Autodesk Inventor part; units mm, degrees
ref_plane "YZ Plane" through (0, 0, 0) normal (1, 0, 0) x (0, 1, 0)
ref_plane "XZ Plane" through (0, 0, 0) normal (0, 1, 0) x (-1, 0, 0)
ref_plane "XY Plane" through (0, 0, 0) normal (0, 0, 1) x (1, 0, 0)
sketch "Sketch1" plane through (0, 0, 0) normal (0, 0, 1) x (1, 0, 0)
  circle A0 centre (0, 0) radius 4.5
  circle A1 centre (0, 0) radius 9.5
  dimension "d0" = 9
  dimension "d1" = 19
extrude "Extrusion1" add sketch "Sketch1" against normal blind 20 contours A0 | A1
extrude "Extrusion2" add sketch "Sketch1" along normal blind 6 contours A0
shell "Shell1" thickness 1.2 removed faces 1 at (2.3703, -2.0999, -20)
chamfer "Chamfer1" distance 5 angle 45 1 edges at (-8.3, 0, -1.2)
properties part number "Marker Plunger" material "ABS Plastic"
Work out the finished part from the listing and answer in its coordinate system (mm). A direction names the side the tool comes from. Give positions to 0.01 mm unless a question says otherwise; leave off trailing zeros. Loops run counter-clockwise (first coordinate to the right, second up) from the corner with the lowest first, then second, coordinate; pieces in that order, holes last. Notation, with made-up numbers: M 53,31 L 90,31 A23 ccw 90,65 Z; hole C 4.5,20.5 d2. An arc over 180 degrees is marked long. Use CSV: the item, a comma, the result in double quotes.
1) Determine the mould class of faces 3 (the cylindrical face through (-0.59, -4.46, 2.96)), 4 (the conical face through (3.446, -1.085, -1.513)), 5 (the flat face through (4.1, 2.2, 0)) for opening direction X: released by +X, released by -X, zero draft, split by the parting line, or undercut.
Answer:
face 3,"split by the parting line"
face 4,"undercut"
face 5,"zero draft"
2) Which of the six approach directions +Z, -Z, +X, -X, +Y, -Y give full straight-line access (tool end or side, diameter ignored) to faces 1 (the cylindrical face through (-1.799, -8.103, -13.003)), 2 (the flat face through (6, -6, -20))?
Answer:
face 1,"-Z"
face 2,"-Z, +X, -X, +Y, -Y"
3) Find section D-D on z = 3. Write down the section's boundary in (x, y), plus the area to 3 significant figures.
Answer:
outline,"C 0,0 d9; hole C 0,0 d6.6"
area,"29.4 mm^2"
4) Given P1, Ø2, axis at y = 4, z = -13.5, coming from the +X side; P2, Ø3.5, axis at x = 1.5, y = -1.5, coming from the -Z side; P3, Ø3, axis at x = -6.5, y = -7, coming from the -Z side; P4, Ø8, axis at x = -2.5, y = -2, coming from the -Z side, each flat-ended and moving along its own axis, determine where each tip first touches the part or whether it passes through.
Answer:
P1,"x = 9.01"
P2,"z = -1.77"
P3,"z = -20"
P4,"z = -5.1"
5) Consider L1, parallel to Y at x = 0, z = 1.55; L2, parallel to Y at x = 0, z = -14.75; L3, parallel to Z at x = 6.25, y = 6.5. Determine where each line is inside the solid, lowest interval first.
Answer:
L1,"-4.5 to -3.3, 3.3 to 4.5"
L2,"-9.5 to -8.3, 8.3 to 9.5"
L3,"-20 to 0"
6) Find section B-B on z = -14.5. Write down the section's boundary in (x, y), plus the area to 3 significant figures.
Answer:
outline,"C 0,0 d19; hole C 0,0 d16.6"
area,"67.1 mm^2"
